Could you check a few things on this model? Use its own coordinates, in mm. Face numbers are marked on the shaded views. A direction names the side the tool comes from. Round coordinates to 2 decimals unless told otherwise and drop trailing zeros. Write each question's results on one line, items separated by ' | '. Start each with the question number.
1) If I drill on probe 1 along X at (y, z) = (26.5, 1.15) (3 decimals); probe 2 along Y at (x, z) = (-1.7, 1.35), over which ranges is the centre line in solid material (lowest first)?
2) Which directions (+Z, -Z, +X, -X, +Y, -Y) give clear straight access to the entire face, cutting with the end or side of a thin tool? Please do the marked faces 1, 2 and 3.
3) For P1, Ø1.1, axis at y = 25, z = 0, coming from the -X side (3 decimals); P2, Ø1.9, axis at y = 25, z = 0, coming from the +X side (3 decimals); P3, Ø1.9, axis at x = 0.5, y = 24.5, coming from the +Z side (3 decimals), each with a flat end and sliding along its axis, tell me the tip position at first contact or that it passes through.
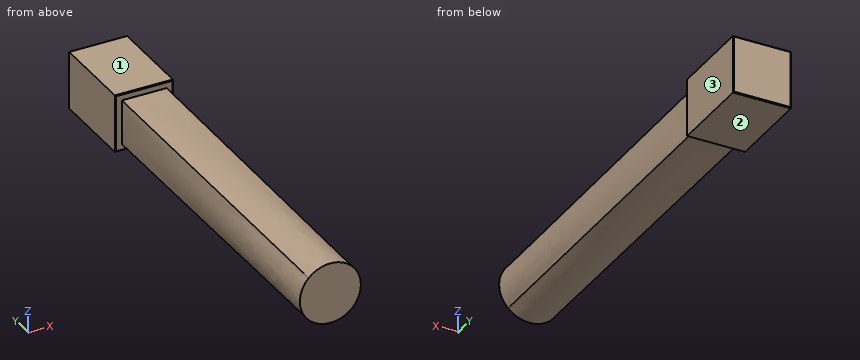
from build123d import *

# Parameters (mm, degrees)
SKETCH3_W           = 3.75
SKETCH3_H           = 3.75
BOSS_EXTRUDE4_DEPTH = 5.6
CHAMFER1_SIZE       = 0.05


with BuildPart() as part:
    # Sketch1 for Loft1 → Loft1 section 0
    with BuildSketch(Plane(origin=(0, 0, 0), x_dir=(1, 0, 0), z_dir=(0, 1, 0))):
        with BuildLine():
            # circular arc as an exact rational Bezier (weights 1, cos(half-angle), 1)
            Bezier((-1.396535893, -1.396535893), (0, -2.793071785), (1.396535893, -1.396535893), weights=[1, 0.707106781, 1])
            Bezier((1.396535893, -1.396535893), (2.793071785, 0), (1.396535893, 1.396535893), weights=[1, 0.707106781, 1])
            Bezier((1.396535893, 1.396535893), (0, 2.793071785), (-1.396535893, 1.396535893), weights=[1, 0.707106781, 1])
            Bezier((-1.396535893, 1.396535893), (-2.793071785, 0), (-1.396535893, -1.396535893), weights=[1, 0.707106781, 1])
        make_face()
    # Sketch2 → Loft1 section 1
    with BuildSketch(Plane(origin=(0, 22.4, 0), x_dir=(1, 0, 0), z_dir=(0, 1, 0))):
        with BuildLine():
            Line((-1.45, -1.45), (1.45, -1.45))
            Line((1.45, -1.45), (1.45, 1.45))
            Line((1.45, 1.45), (-1.45, 1.45))
            Line((-1.45, 1.45), (-1.45, -1.45))
        make_face()
    loft()

    # Sketch3 → Boss-Extrude4 (add)
    with BuildSketch(Plane(origin=(0, 22.4, 0), x_dir=(1, 0, 0), z_dir=(0, 1, 0))):
        Rectangle(SKETCH3_W, SKETCH3_H)
    extrude(amount=BOSS_EXTRUDE4_DEPTH)

    # Chamfer1
    chamfer1_edges = [part.edges().sort_by_distance(p)[0] for p in [
        (1.875, 22.4, 0),
        (0, 22.4, -1.875),
        (-1.875, 22.4, 0),
        (0, 22.4, 1.875),
        (1.875, 28, 0),
        (0, 28, -1.875),
        (-1.875, 28, 0),
        (0, 28, 1.875),
    ]]
    chamfer(chamfer1_edges, length=CHAMFER1_SIZE)


solid = part.part
Checked values:
1) probe 1: -1.875 to 1.875 | probe 2: 22.4 to 28
2) face 1: +Z, +X, -X, +Y | face 2: -Z, +X, -X, +Y | face 3: +Z, -Z, +X, +Y
3) P1: x = -1.875 | P2: x = 1.875 | P3: z = 1.875
